Could you check a few things on this model? Use its own coordinates, in mm. Give positions to 0.01 mm unless a question says otherwise; leave off trailing zeros. Order: outer loops, then holes, each group sorted by start corner. A loop starts at its lowest first (then second) coordinate and runs counter-clockwise, first axis right, second up. Notation, with made-up numbers: (35, 11) -> (93, 11) arc R23 ccw to (93, 20) -> close; hole circle Ø5 at (78.25, 26.5). An arc over 180 degrees is marked (long way). Answer as CSV lines item,"result". Start each with the question number.
(1) I want a section at A-A (z = 2.25). Please give me the cut outline in (x, y).
(2) We'd pull the mould along X, two halves only. Please class faces 1 (the face through (4.77, -1.5, 2.26)), 2 (the face through (0.3, -5.2, 0)): released by +X, released by -X, zero draft, split by the parting line, or undercut.
(3) Will these pins go through, and if not, where does the flat tip stop? pin 1 Ø5 at (y, z) = (14, 3.5) entering from +X; pin 2 Ø2 at (y, z) = (13, 11.5) entering from -X; pin 3 Ø5 at (y, z) = (-5.5, 9.5) entering from -X.
(4) I need wall thicknesses on L1, parallel to X at y = -4, z = 10.25; L2, parallel to Y at x = 0, z = 2.5; L3, parallel to X at y = 0, z = 2.2. Which ranges of each line are inside material? Lowest first, please.
(5) I want a section at B-B (z = 6). Please give me the cut outline in (x, y), plus the area to 3 significant figures.
```python
from build123d import *

# Parameters (mm, degrees)
F2_R = 1


with BuildPart() as f1:
    # F0 (on Front) → F1 (revolve)
    with BuildSketch(Plane.XZ):
        with BuildLine():
            ThreePointArc((20, 0), (18.4775906502, 7.6536686473), (14.1421356237, 14.1421356237))
            Line((14.1421356237, 14.1421356237), (5, 5))
            Line((5, 5), (5, 0))
            Line((5, 0), (20, 0))
        make_face()
    revolve(axis=Axis((0, 0, 1.4953076416), (0, 0, -1)))

    # F2
    f2_edges = [f1.edges().sort_by_distance(p)[0] for p in [
        (-5, 0, 5),
        (-14.142136, 0, 14.142136),
        (-20, 0, 0),
    ]]
    fillet(f2_edges, radius=F2_R)


solid = f1.part
```
Final values:
1,outline,"circle Ø39.75 at (0, 0); hole circle Ø10 at (0, 0)"
2,face 1,"undercut"
2,face 2,"zero draft"
3,pin 1,"x = 16.05"
3,pin 2,"x = -11.51"
3,pin 3,"x = -18.11"
4,L1,"-16.7 to -9.44, 9.44 to 16.7"
4,L2,"-19.84 to -5, 5 to 19.84"
4,L3,"-19.88 to -5, 5 to 19.88"
5,outline,"circle Ø38.16 at (0, 0); hole circle Ø12 at (0, 0)"
5,area,"1,030 mm²"
